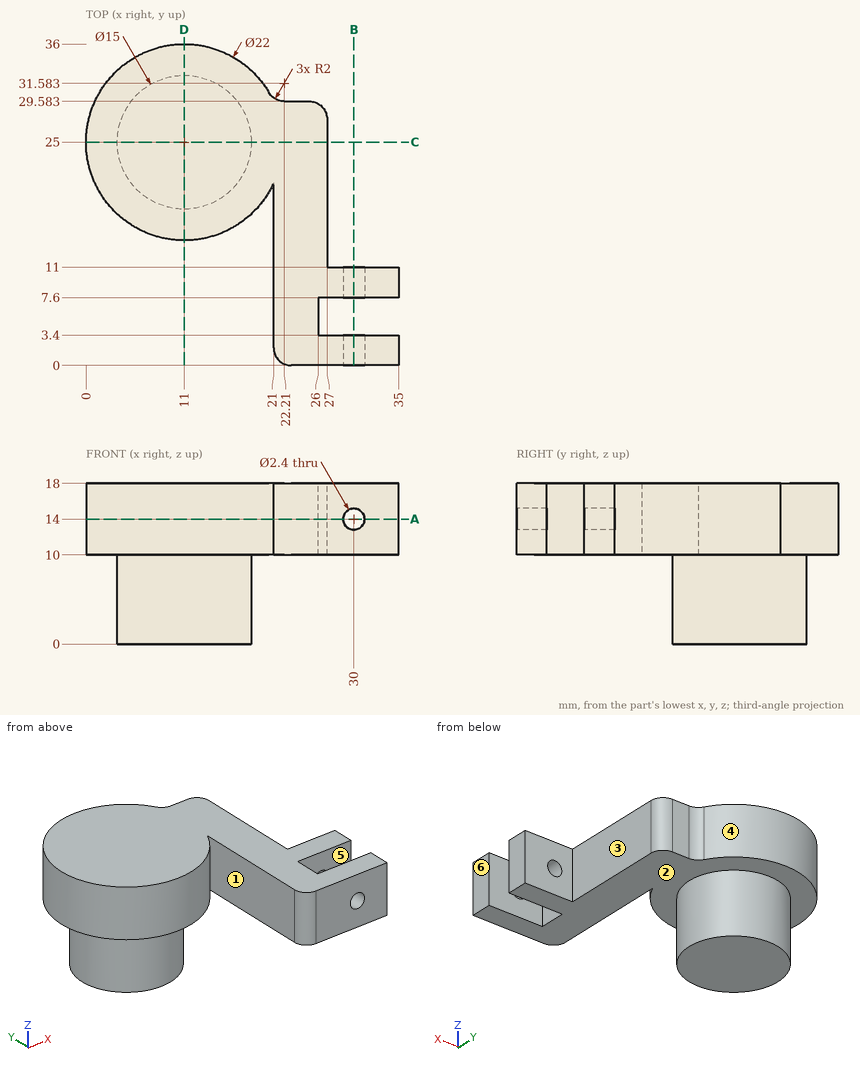
Input: dimensioned drawing with shaded views. Units: mm. Origin: part minimum x, y, z. A direction names the side the tool comes from. Give positions to 0.01 mm unless a question says otherwise; leave off trailing zeros. Write each loop counter-clockwise with the first axis right and the second up, starting at its lowest first coordinate (ties: lowest second). Pieces come first, ordered by that corner, then holes.
Q1. Set-up query: the marked faces 1, 2 and 3. Return all of +Z, -Z, +X, -X, +Y, -Y with unobstructed straight access to the full face (end or side cutting, diameter ignored); none if empty.
Q2. First-contact query: P1, Ø6.5, axis at x = 29.5, z = 15, coming from the +Y side (1 decimal); P2, Ø6, axis at x = 26.5, z = 4.5, coming from the +Y side; P3, Ø9, axis at x = 32.5, z = 15.5, coming from the +Y side; P4, Ø4, axis at y = 31.5, z = 10.5, coming from the -X side. Flat tips, straight axial feed; report the tip coordinate or a pass-through.
Q3. Section B-B, the plane x = 30. Output: boundary loops of the cut face in (y, z).
Q4. Section C-C, the plane y = 25. Output: boundary loops of the cut face in (x, z), plus the area to 3 significant figures.
Q5. Section D-D, the plane x = 11. Output: boundary loops of the cut face in (y, z).
Q6. Section A-A, the plane z = 14. Output: boundary loops of the cut face in (x, y) (1 decimal), plus the area to 3 significant figures.
Q7. Pull-direction query (X, two-part tool) for the marked faces 4, 5 and 6; classes: pulls with the +X half, pulls with the -X half, needs draft (parallel to the pull), parting line crosses it, or undercut.
Q8. Material intervals for probe 1 along Z at (x, y) = (30, 1.9); probe 2 along Y at (x, z) = (11, 12.75); probe 3 along Z at (x, y) = (24, 11.5), sorted ascending.
Filled in:
1. face 1: +Z, -Z, -Y
1. face 2: -Z
1. face 3: +Z, -Z, +X, +Y
2. P1: stops at y = 29.1
2. P2: passes through
2. P3: stops at y = 11
2. P4: stops at x = 0.96
3. outline: (0, 10) - (3.4, 10) - (3.4, 12.8) - (0, 12.8) - close; (0, 15.2) - (3.4, 15.2) - (3.4, 18) - (0, 18) - close; (7.6, 10) - (11, 10) - (11, 12.8) - (7.6, 12.8) - close; (7.6, 15.2) - (11, 15.2) - (11, 18) - (7.6, 18) - close
4. outline: (0, 10) - (3.5, 10) - (3.5, 0) - (18.5, 0) - (18.5, 10) - (27, 10) - (27, 18) - (0, 18) - close
4. area: 366 mm2
5. outline: (14, 10) - (17.5, 10) - (17.5, 0) - (32.5, 0) - (32.5, 10) - (36, 10) - (36, 18) - (14, 18) - close
6. outline: (20.5, 30.6) arc R11 ccw (long way) to (21, 20.4) - (21, 2) arc R2 ccw to (23, 0) - (28.8, 0) - (28.8, 3.4) - (26, 3.4) - (26, 7.6) - (28.8, 7.6) - (28.8, 11) - (27, 11) - (27, 27.6) arc R2 ccw to (25, 29.6) - (22.2, 29.6) arc R2 cw to start; (31.2, 0) - (35, 0) - (35, 3.4) - (31.2, 3.4) - close; (31.2, 7.6) - (35, 7.6) - (35, 11) - (31.2, 11) - close
6. area: 584 mm2
7. face 4: undercut
7. face 5: needs draft
7. face 6: pulls with the +X half
8. probe 1: z = 10 to 12.8, 15.2 to 18
8. probe 2: y = 14 to 36
8. probe 3: z = 10 to 18
